from build123d import *

# Parameters (mm, degrees)
SKETCH1_W           = 53.26
SKETCH1_H           = 39.29
BOSS_EXTRUDE1_DEPTH = 5
FILLET1_R           = 2
SKETCH2_R           = 2.55
CUT_EXTRUDE1_DEPTH  = 4.1
SKETCH3_W           = 2
SKETCH3_H           = 9
BOSS_EXTRUDE2_DEPTH = 4


with BuildPart() as part:
    # Sketch1 → Boss-Extrude1 (new body)
    with BuildSketch(Plane(origin=(0, 0, 0), x_dir=(1, 0, 0), z_dir=(0, 1, 0))):
        Rectangle(SKETCH1_W, SKETCH1_H)
    extrude(amount=BOSS_EXTRUDE1_DEPTH)

    # Fillet1
    fillet1_edges = [part.edges().sort_by_distance(p)[0] for p in [
        (26.63, 2.5, 19.645),
        (-26.63, 2.5, 19.645),
        (-26.63, 2.5, -19.645),
        (26.63, 2.5, -19.645),
    ]]
    fillet(fillet1_edges, radius=FILLET1_R)

    # Sketch2 → Cut-Extrude1 (cut)
    with BuildSketch(Plane(origin=(0, 0, 0), x_dir=(-1, 0, 0), z_dir=(0, -1, 0))):
        with Locations(Location((23.03, -16.045, 0), (0, 0, 90))):
            Circle(SKETCH2_R)
        with Locations(Location((23.03, 16.045, 0), (0, 0, 90))):
            Circle(SKETCH2_R)
    extrude(amount=-CUT_EXTRUDE1_DEPTH, mode=Mode.SUBTRACT)

    # Sketch3 → Boss-Extrude2 (add)
    with BuildSketch(Plane(origin=(0, 0, 0), x_dir=(-1, 0, 0), z_dir=(0, -1, 0))):
        with Locations((-25.63, -2.748)):
            Rectangle(SKETCH3_W, SKETCH3_H)
    extrude(amount=BOSS_EXTRUDE2_DEPTH)


solid = part.part
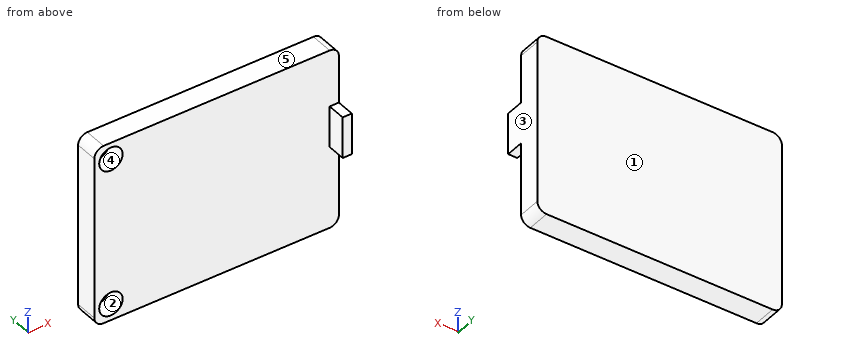
The listing builds one solid part. Answer for the finished solid, in the listing's coordinates (mm). Face numbers are marked on the shaded views. A direction names the side the tool comes from. Round coordinates to 2 decimals unless told otherwise and drop trailing zeros. Write each loop counter-clockwise with the first axis right and the second up, starting at its lowest first coordinate (ties: lowest second). Pieces come first, ordered by that corner, then holes. Notation, with made-up numbers: M 56.5,-12 L 105.5,-12 A4 cw 105.5,-5 Z; hole C -18,9 d10. An arc over 180 degrees is marked long. Write each question's results on one line, items separated by ' | '. Start each with the question number.
Item 1: Given pin 1 Ø2 at (y, z) = (-2, 4.5) entering from -X; pin 2 Ø1.6 at (x, y) = (25.5, -2.5) entering from +Z; pin 3 Ø2.5 at (x, z) = (-22, 16.5) entering from -Y, each flat-ended and moving along its own axis, determine where each tip first touches the part or whether it passes through.
Item 2: Find section C-C on z = 3. Write down the section's boundary in (x, y), and give its area (3 significant figures).
Item 3: Find section D-D on y = -2.75. Write down the section's boundary in (x, z).
Item 4: The mould has two halves that part along X. Classify the marked faces 1, 2 and 3: +X half, -X half, draft (parallel to the pull), parting line (faces both ways), or undercut.
Item 5: Find section B-B on y = 1.25. Write down the section's boundary in (x, z) (3 decimals).
Item 6: Which of the six approach directions +Z, -Z, +X, -X, +Y, -Y give full straight-line access (tool end or side, diameter ignored) to the marked faces 4 and 5?
Item 7: Straight lines are drawn through the part: probe 1 along Z at (x, y) = (-21.5, 1) (3 decimals); probe 2 along Y at (x, z) = (8, 0); probe 3 along Y at (x, z) = (-22, 14.5). For each, find the intervals that lie inside material, in ascending order.
Item 8: Find section A-A on x = -23.03. Write down the section's boundary in (y, z) (3 decimals).
Answer block:
1) pin 1: stops at x = 24.63 | pin 2: stops at z = 7.25 | pin 3: stops at y = 4.1
2) outline: M -26.63,0 L 24.63,0 L 24.63,-4 L 26.63,-4 L 26.63,5 L -26.63,5 Z | area: 274 mm²
3) outline: M 24.63,-1.75 L 26.63,-1.75 L 26.63,7.25 L 24.63,7.25 Z
4) face 1: draft | face 2: undercut | face 3: +X half
5) outline: M -26.63,-17.645 A2 ccw -24.63,-19.645 L 24.63,-19.645 A2 ccw 26.63,-17.645 L 26.63,17.645 A2 ccw 24.63,19.645 L -24.63,19.645 A2 ccw -26.63,17.645 Z; hole C -23.03,-16.045 d5.1; hole C -23.03,16.045 d5.1
6) face 4: -Y | face 5: +Z, +X, -X, +Y, -Y
7) probe 1: z = -19.645 to -18.085, -14.005 to 14.005, 18.085 to 19.645 | probe 2: y = 0 to 5 | probe 3: y = 4.1 to 5
8) outline: M 0,-19.645 L 5,-19.645 L 5,19.645 L 0,19.645 L 0,18.595 L 4.1,18.595 L 4.1,13.495 L 0,13.495 L 0,-13.495 L 4.1,-13.495 L 4.1,-18.595 L 0,-18.595 Z
